Source: three-view drawing plus pictorial views. Frame: mm from the lowest corner of the part. Give positions to 0.01 mm unless a question says otherwise; leave off trailing zeros. Order: outer loops, then holes, each group sorted by start corner. A loop starts at its lowest first (then second) coordinate and runs counter-clockwise, first axis right, second up. Notation, with made-up numbers: (18, -7.5) - (74, -7.5) arc R33 cw to (74, 28.5) - close; hole circle Ø7 at (-40, 70.5). An arc over 180 degrees is marked (long way). Use CSV: the item, a comma, the result in double quotes.
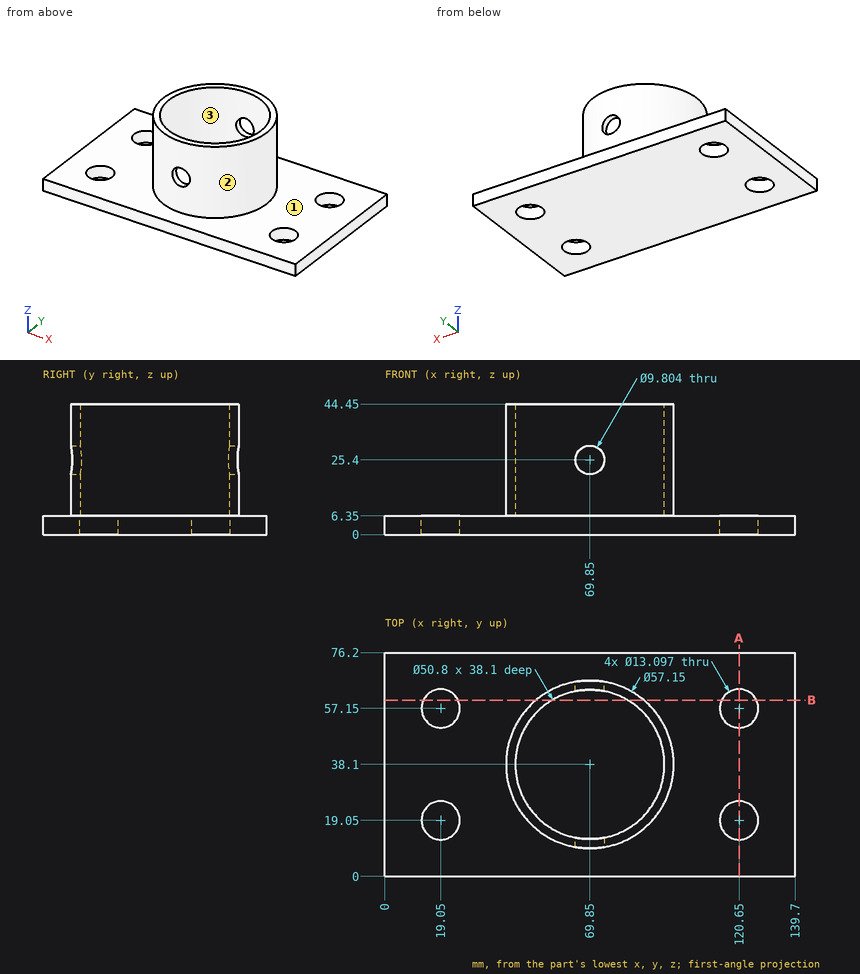
Item 1: First-contact query: pin 1 (6 mm diameter, centred on x = 69.85, z = 25.4, fed in from +Y); pin 2 (21 mm diameter, centred on x = 19.05, y = 19.05, fed in from +Z); pin 3 (4 mm diameter, centred on y = 19, z = 20, fed in from +X) (1 decimal); pin 4 (8 mm diameter, centred on x = 99.5, z = 15.5, fed in from +Y) (1 decimal). Flat tips, straight axial feed; report the tip coordinate or a pass-through.
Filled in:
pin 1,"passes through"
pin 2,"stops at z = 6.35"
pin 3,"stops at x = 92.7"
pin 4,"stops at y = 50.7"
Item 2: Material intervals for line 1 (X direction, y = 19.05, z = 3.75); line 2 (Y direction, x = 120.65, z = 5.25); line 3 (Z direction, x = 69.85, y = 10.45), sorted ascending. Write a range as from..to.
Filled in:
line 1,"x = 0..12.5, 25.6..114.1, 127.2..139.7"
line 2,"y = 0..12.5, 25.6..50.6, 63.7..76.2"
line 3,"z = 0..20.5, 30.3..44.45"
Item 3: Mould query, pull axis Y, two halves, no side actions, for the marked faces 1, 2 and 3. Classes: released by +Y, released by -Y, zero draft, split by the parting line, or undercut.
Filled in:
face 1,"zero draft"
face 2,"split by the parting line"
face 3,"undercut"
Item 4: Section A-A on x = 120.65. Return the cut outline in (y, z).
Filled in:
outline,"(0, 0) - (12.5, 0) - (12.5, 6.35) - (0, 6.35) - close; (25.6, 0) - (50.6, 0) - (50.6, 6.35) - (25.6, 6.35) - close; (63.7, 0) - (76.2, 0) - (76.2, 6.35) - (63.7, 6.35) - close"
Item 5: Section B-B on y = 60. Count the separate pieces of the cut face and the enclosed holes in it, then the cut area to 3 significant figures.
Filled in:
separate pieces,"3"
enclosed holes,"0"
area,"1,160 mm2"
